Read the model definition and answer for the solid it produces. Units are mm, in the model's axes. Give positions to 0.01 mm unless a question says otherwise; leave off trailing zeros. Write each loop counter-clockwise with the first axis right and the second up, starting at its lowest first coordinate (ties: lowest second). Pieces come first, ordered by that corner, then holes.
```python
from build123d import *

# Parameters (mm, degrees)
BOSS_EXTRUDE1_DEPTH = 16
CUT_EXTRUDE2_DEPTH  = 2104.387610499
SKETCH6_W           = 32
SKETCH6_H           = 32
SKETCH6_H_2         = 26
CUT_EXTRUDE4_DEPTH  = 1063.402282565


with BuildPart() as part:
    # Sketch1 → Boss-Extrude1 (new body)
    with BuildSketch(Plane.XY):
        Polygon((173, 1048.1), (-173, 915.283043878), (-173, -1048.1), (173, -1048.1), align=None)
    extrude(amount=BOSS_EXTRUDE1_DEPTH)

    # Sketch3 → Cut-Extrude2 (cut, through all)
    with BuildSketch(Plane.XZ.offset(1048.1)):
        Polygon((-173, 16), (-157, 0), (-173, 0), align=None)
    extrude(amount=-CUT_EXTRUDE2_DEPTH, mode=Mode.SUBTRACT)

    # Sketch6 → Cut-Extrude4 (cut, through all)
    with BuildSketch(Plane.XY.offset(16)):
        with Locations((157, 1000.1)):
            Rectangle(SKETCH6_W, SKETCH6_H)
        with Locations((157, -1000.1)):
            Rectangle(SKETCH6_W, SKETCH6_H)
        with Locations((157, -944.1)):
            Rectangle(SKETCH6_W, SKETCH6_H_2)
    extrude(amount=-CUT_EXTRUDE4_DEPTH, mode=Mode.SUBTRACT)


solid = part.part
```
Item 1: Determine the mould class of faces 1 (the flat face through (-2, 15, 16)), 2 (the flat face through (2.42, 982.62, 7.89)) for opening direction Y: pulls with the +Y half, pulls with the -Y half, needs draft (parallel to the pull), parting line crosses it, or undercut.
Result set:
face 1: needs draft
face 2: pulls with the +Y half
Item 2: Each of these flat-tipped pins is pushed along its axis until it touches: pin 1 Ø10 at (x, y) = (60, 120.5) entering from -Z; pin 2 Ø8 at (x, z) = (149.5, 11.5) entering from +Y; pin 3 Ø5 at (x, z) = (-83, 8.5) entering from +Y; pin 4 Ø1.5 at (x, z) = (-14.5, 5) entering from +Y. Where does it stop, or does it pass through?
Result set:
pin 1: stops at z = 0
pin 2: stops at y = 1040.61
pin 3: stops at y = 950.79
pin 4: stops at y = 976.41
Item 3: Section C-C (x = 26) is taken. Write down the section's boundary in (y, z).
Result set:
outline: (-1048.1, 0) - (991.67, 0) - (991.67, 16) - (-1048.1, 16) - close
Item 4: Section A-A (z = 7.75) is taken. Write down the section's boundary in (x, y).
Result set:
outline: (-164.75, -1048.1) - (173, -1048.1) - (173, -1016.1) - (141, -1016.1) - (141, -984.1) - (173, -984.1) - (173, -957.1) - (141, -957.1) - (141, -931.1) - (173, -931.1) - (173, 984.1) - (141, 984.1) - (141, 1016.1) - (173, 1016.1) - (173, 1048.1) - (-164.75, 918.45) - close
Item 5: Section B-B (y = 497.5) is taken. Write down the section's boundary in (x, z).
Result set:
outline: (-173, 16) - (-157, 0) - (173, 0) - (173, 16) - close
Item 6: Find the intervals of material crossed by line 1 along Y through (x, z) = (151, 4.75) (3 decimals); line 2 along Y through (x, z) = (25, 4); line 3 along Y through (x, z) = (-152.5, 5.5), in increasing order.
Result set:
line 1: y = -1048.1 to -1016.1, -984.1 to -957.1, -931.1 to 984.1, 1016.1 to 1039.655
line 2: y = -1048.1 to 991.29
line 3: y = -1048.1 to 923.15
